```python
from build123d import *

# Parameters (mm, degrees)
SKETCH1_R           = 10.287
BOSS_EXTRUDE1_DEPTH = 3.175
SKETCH2_R           = 4.8514
BOSS_EXTRUDE2_DEPTH = 288.925
SKETCH3_R           = 4.064
CUT_EXTRUDE1_DEPTH  = 1.27
FILLET1_R           = 1.000000032
CUT_EXTRUDE2_REACH  = 294.462
SKETCH4_R           = 1.27
CIRPATTERN1_COUNT   = 4
FILLET2_R           = 3.81


with BuildPart() as part:
    # Sketch1 → Boss-Extrude1 (new body)
    with BuildSketch(Plane.XY):
        Circle(SKETCH1_R)
    extrude(amount=BOSS_EXTRUDE1_DEPTH)

    # Sketch2 → Boss-Extrude2 (add)
    with BuildSketch(Plane.XY.offset(3.175)):
        Circle(SKETCH2_R)
    extrude(amount=BOSS_EXTRUDE2_DEPTH)

    # Sketch3 → Cut-Extrude1 (cut)
    with BuildSketch(Plane(origin=(0, 0, 0), x_dir=(-1, 0, 0), z_dir=(0, 0, -1))):
        Circle(SKETCH3_R)
    extrude(amount=-CUT_EXTRUDE1_DEPTH, mode=Mode.SUBTRACT)

    # Fillet1
    fillet1_edges = [part.edges().sort_by_distance(p)[0] for p in [
        (4.064, 0, 0),
    ]]
    fillet(fillet1_edges, radius=FILLET1_R)

    # Sketch4 → Cut-Extrude2 (cut, up to next)
    with BuildSketch(Plane(origin=(0, 0, 0), x_dir=(-1, 0, 0), z_dir=(0, 0, -1)), mode=Mode.PRIVATE) as cut_extrude2_sk1:
        with Locations((0, 7.874)):
            Circle(SKETCH4_R)
    cut_extrude2_tool1 = extrude(cut_extrude2_sk1.sketch, amount=-CUT_EXTRUDE2_REACH, mode=Mode.PRIVATE) & part.part
    cut_extrude2 = cut_extrude2_tool1.solids().sort_by_distance((0, 7.874, 0))[0]
    add(cut_extrude2, mode=Mode.SUBTRACT)

    # CirPattern1: Cut-Extrude2 ×4 about axis
    cirpattern1_axis = Axis((0, 0, 0), (0, 0, 1))
    for i in range(1, CIRPATTERN1_COUNT):
        add(cut_extrude2.rotate(cirpattern1_axis, i * 360 / CIRPATTERN1_COUNT), mode=Mode.SUBTRACT)

    # Fillet2
    # the kernel refuses this fillet: 3.81 mm, written as the material it adds along each edge
    with BuildSketch(Plane(origin=(0, 0, 3.175), x_dir=(1, 0, 0), z_dir=(0, -1, 0))) as fillet2_piece_1_section:
        with BuildLine():
            CenterArc((4.8514 + FILLET2_R, FILLET2_R), FILLET2_R, 180, 90)
            Line((4.8514, FILLET2_R), (4.8514, 0))
            Line((4.8514, 0), (4.8514 + FILLET2_R, 0))
        make_face()
    fillet2_piece_1 = revolve(axis=Axis((0, 0, 3.175), (0, 0, 1)), mode=Mode.PRIVATE)
    fillet2_piece_1 = fillet2_piece_1 - Plane(origin=(-7.874, 0, 4.25520668), x_dir=(0, -1, 0), z_dir=(0, 0, -1)) * Cylinder(1.27, 35, mode=Mode.PRIVATE)
    fillet2_piece_1 = fillet2_piece_1 - Plane(origin=(0, -7.874, 4.25520668), x_dir=(1, 0, 0), z_dir=(0, 0, -1)) * Cylinder(1.27, 35, mode=Mode.PRIVATE)
    fillet2_piece_1 = fillet2_piece_1 - Plane(origin=(0, 7.874, 4.25520668), x_dir=(-1, 0, 0), z_dir=(0, 0, -1)) * Cylinder(1.27, 35, mode=Mode.PRIVATE)
    fillet2_piece_1 = fillet2_piece_1 - Plane(origin=(7.874, 0, 4.25520668), x_dir=(0, 1, 0), z_dir=(0, 0, -1)) * Cylinder(1.27, 35, mode=Mode.PRIVATE)
    add(fillet2_piece_1)


solid = part.part
```
Verification items for the finished model (mm, model axes). Coordinates: 2 decimals unless noted, no trailing zeros. Loops run counter-clockwise (first coordinate to the right, second up) from the corner with the lowest first, then second, coordinate; pieces in that order, holes last. Notation, with made-up numbers: (82, -2) -> (90, -2) arc R18 ccw to (90, 21) -> close; hole circle Ø10 at (51, -8.75). An arc over 180 degrees is marked (long way). Answer in a Markdown table with one row per item.
1) Draft check along Y on faces 1 (the face through (-5, 8, 3.175)), 2 (the face through (0, 0, 1.27)), 3 (the face through (4.627, 1.457, 147.547)). Enter one of: released by +Y, released by -Y, zero draft, split by the parting line, or undercut.
The answers:
| item | result |
|---|---|
| face 1 | zero draft |
| face 2 | undercut |
| face 3 | split by the parting line |
2) Depth check by flat-ended pin: P1, Ø4, axis at x = 1, y = 0.5, coming from the -Z side; P2, Ø4, axis at x = 0, y = -7.874, coming from the +Z side; P3, Ø5, axis at y = 4, z = 184, coming from the +X side. Enter the tip coordinate at first touch or a pass-through.
The answers:
| item | result |
|---|---|
| P1 | stops at z = 1.27 |
| P2 | stops at z = 4.39 |
| P3 | stops at x = 4.61 |
3) Scan lines: line 1 along Y through (x, z) = (0, 2.4); line 2 along Y through (x, z) = (0, 1.1); line 3 along Z through (x, y) = (8, 5.75) (3 decimals). Record each from-to range of solid material in increasing order. Write a range as from..to.
The answers:
| item | result |
|---|---|
| line 1 | y = -10.29..-9.14, -6.6..6.6, 9.14..10.29 |
| line 2 | y = -10.29..-9.14, -6.6..-4.06, 4.06..6.6, 9.14..10.29 |
| line 3 | z = 0..3.175 |
4) Section check A-A (z = 68.5). Record the cut outline in (x, y).
The answers:
| item | result |
|---|---|
| outline | circle Ø9.7 at (0, 0) |
